Check sheet for the modelled part. Datum: model origin and axes. Units: mm. Give positions to 0.01 mm unless a question says otherwise; leave off trailing zeros. Order: outer loops, then holes, each group sorted by start corner. A loop starts at its lowest first (then second) coordinate and runs counter-clockwise, first axis right, second up.
```python
from build123d import *

# Parameters (mm, degrees)
F0_R     = 6.35
F1_DEPTH = 12.7


with BuildPart() as f1:
    # F0 (on Top) → F1 (new body)
    with BuildSketch(Plane.XY):
        with BuildLine():
            Line((35.025607, 17.338161), (-35.143936, 17.338161))
            Line((-35.143936, 17.338161), (-16.562536, -8.254128))
            ThreePointArc((-16.562536, -8.254128), (-12.053122, -12.1074), (-6.285636, -13.492538))
            Line((-6.285636, -13.492538), (6.167308, -13.492538))
            ThreePointArc((6.167308, -13.492538), (11.934794, -12.1074), (16.444207, -8.254128))
            Line((16.444207, -8.254128), (35.025607, 17.338161))
        make_face()
        Circle(F0_R, mode=Mode.SUBTRACT)
    extrude(amount=F1_DEPTH)


solid = f1.part
```
(1) Sectioned sample at C-C (y = 0). Enter the section's corners in (x, z).
(2) Thickness scan on L1, parallel to Y at x = 0, z = 10; L2, parallel to Y at x = 6.5, z = 12; L3, parallel to Y at x = 3.5, z = 3. Record the ranges inside material, lowest first.
(3) Release check for a two-part mould opening along Y. For faces 1 (the face through (25.605, 4.363, 6.261)), 2 (the face through (-1, 9, 0)), 3 (the face through (-1.38, -6.2, 6.26)) record: released by +Y, released by -Y, zero draft, split by the parting line, or undercut.
(4) Go/stop test with flat-tipped pins: P1, Ø1, axis at y = 9.5, z = 1.5, coming from the -X side; P2, Ø1, axis at x = -17.5, y = -8.5, coming from the +Z side; P3, Ø6, axis at y = 1.5, z = 8.5, coming from the +X side. Record where each tip stops, or that it passes through.
(5) Sectioned sample at A-A (x = 0). Enter the section's corners in (y, z), plus the area to 3 significant figures.
(6) Sectioned sample at D-D (x = -20). Enter the section's corners in (y, z), plus the area to 3 significant figures.
(7) Sectioned sample at B-B (z = 1.5). Enter the section's corners in (x, y).
Values follow:
1. outline: (-22.56, 0) - (-6.35, 0) - (-6.35, 12.7) - (-22.56, 12.7) - close; (6.35, 0) - (22.44, 0) - (22.44, 12.7) - (6.35, 12.7) - close
2. L1: y = -13.49 to -6.35, 6.35 to 17.34
2. L2: y = -13.49 to 17.34
2. L3: y = -13.49 to -5.3, 5.3 to 17.34
3. face 1: released by -Y
3. face 2: zero draft
3. face 3: undercut
4. P1: stops at x = -29.82
4. P2: passes through
4. P3: stops at x = 25.7
5. outline: (-13.49, 0) - (-6.35, 0) - (-6.35, 12.7) - (-13.49, 12.7) - close; (6.35, 0) - (17.34, 0) - (17.34, 12.7) - (6.35, 12.7) - close
5. area: 230 mm2
6. outline: (-3.52, 0) - (17.34, 0) - (17.34, 12.7) - (-3.52, 12.7) - close
6. area: 265 mm2
7. outline: (-35.14, 17.34) - (-16.56, -8.25) arc R12.7 ccw to (-6.29, -13.49) - (6.17, -13.49) arc R12.7 ccw to (16.44, -8.25) - (35.03, 17.34) - close; hole circle Ø12.7 at (0, 0)
